Read the model definition and answer for the solid it produces. Units are mm, in the model's axes. A direction names the side the tool comes from. Give positions to 0.01 mm unless a question says otherwise; leave off trailing zeros. Write each loop counter-clockwise with the first axis right and the second up, starting at its lowest first coordinate (ties: lowest second). Pieces come first, ordered by that corner, then holes.
```python
from build123d import *

# Parameters (mm, degrees)
BOSS_EXTRUDE1_DEPTH = 3.175
SKETCH2_W           = 1.27
SKETCH2_H           = 5.08
SKETCH2_W_2         = 12.7
SKETCH2_H_2         = 8.89
CUT_EXTRUDE1_DEPTH  = 3.175


with BuildPart() as part:
    # Sketch1 → Boss-Extrude1 (new body)
    with BuildSketch(Plane(origin=(0, 0, 0), x_dir=(1, 0, 0), z_dir=(0, 1, 0))):
        Polygon((32.661869368, 101.6), (127, 101.6), (127, 0), (-127, 0), (-127, 101.6), (-32.661869368, 101.6), (-53.975, 76.2), (53.975, 76.2), align=None)
    extrude(amount=BOSS_EXTRUDE1_DEPTH)

    # Sketch2 → Cut-Extrude1 (cut)
    with BuildSketch(Plane(origin=(0, 3.175, 0), x_dir=(-1, 0, 0), z_dir=(0, 1, 0))):
        with Locations((38.735, -73.66)):
            Rectangle(SKETCH2_W, SKETCH2_H)
        Polygon((52.3875, -72.39), (49.190530405, -76.2), (53.975, -76.2), (51.310858671, -79.375), (55.5625, -79.375), (55.5625, -72.39), align=None)
        Polygon((12.7, -76.2), (15.24, -76.2), (15.24, -59.055), (13.97, -59.055), (13.97, -71.12), (12.7, -71.12), align=None)
        with Locations((0, -71.755)):
            Rectangle(SKETCH2_W_2, SKETCH2_H_2)
        with Locations((-13.335, -73.66)):
            Rectangle(SKETCH2_W, SKETCH2_H)
        with Locations((-38.735, -73.66)):
            Rectangle(SKETCH2_W, SKETCH2_H)
        Polygon((-53.975, -76.2), (-49.190530405, -76.2), (-52.3875, -72.39), (-55.5625, -72.39), (-55.5625, -79.375), (-51.310858671, -79.375), align=None)
    extrude(amount=-CUT_EXTRUDE1_DEPTH, mode=Mode.SUBTRACT)


solid = part.part
```
Item 1: Determine the mould class of faces 3 (the flat face through (42.12, 1.57, -90.33)), 4 (the flat face through (2, 3.175, -52)) for opening direction X: pulls with the +X half, pulls with the -X half, needs draft (parallel to the pull), parting line crosses it, or undercut.
Result set:
face 3: undercut
face 4: needs draft
Item 2: Which of the six approach directions +Z, -Z, +X, -X, +Y, -Y give full straight-line access (tool end or side, diameter ignored) to faces 1 (the flat face through (-41.86, 1.57, -90.64)), 2 (the flat face through (2, 0, -52))?
Result set:
face 1: +Y, -Y
face 2: +Z, -Z, +X, -X, -Y
Item 3: Each of these flat-tipped pins is pushed along its axis until it touches: pin 1 Ø1 at (x, y) = (-45.5, 0.5) entering from +Z; pin 2 Ø0.6 at (x, y) = (-15, 2) entering from -Z; pin 3 Ø1 at (x, y) = (-13.5, 1.5) entering from -Z. Where does it stop, or does it pass through?
Result set:
pin 1: stops at z = 0
pin 2: stops at z = -76.2
pin 3: stops at z = -71.12
Item 4: Find the intervals of material crossed by line 1 along X through (y, z) = (1, -69); line 2 along X through (y, z) = (0.4, -77); line 3 along Z through (x, y) = (-10.5, 2.55), in increasing order.
Result set:
line 1: x = -127 to -15.24, -13.97 to -6.35, 6.35 to 127
line 2: x = -127 to -55.56, 55.56 to 127
line 3: z = -76.2 to 0
Item 5: Section A-A (x = 35) is taken. Write down the section's boundary in (y, z) (3 decimals), and give its area (3 significant figures).
Result set:
outline: (0, -101.6) - (3.175, -101.6) - (3.175, -98.814) - (0, -98.814) - close; (0, -76.2) - (3.175, -76.2) - (3.175, 0) - (0, 0) - close
area: 251 mm2
Item 6: Section C-C (x = -18) is taken. Write down the section's boundary in (y, z) (3 decimals).
Result set:
outline: (0, -76.2) - (3.175, -76.2) - (3.175, 0) - (0, 0) - close
Item 7: Section B-B (z = -86.5) is taken. Write down the section's boundary in (x, y) (3 decimals), and give its area (3 significant figures).
Result set:
outline: (-127, 0) - (-45.332, 0) - (-45.332, 3.175) - (-127, 3.175) - close; (45.332, 0) - (127, 0) - (127, 3.175) - (45.332, 3.175) - close
area: 519 mm2
